from build123d import *

# Parameters (mm, degrees)
F1_DEPTH = 40
F2_W     = 40
F2_H     = 20
F3_DEPTH = 40.001
F4_R     = 5


with BuildPart() as f1:
    # F0 (on Right) → F1 (new body)
    with BuildSketch(Plane.YZ):
        Polygon((-151.999998, 380), (-184, 0), (-143.858423, 0), (-137.725254, 72.831372), (148.000002, 72.831372), (148.000002, 0), (188.000002, 0), (188.000002, 680), (163.722336, 680), (148.000002, 380), align=None)
        Polygon((148.000002, 112.831372), (-134.356833, 112.831372), (-115.226841, 340), (148.000002, 340), align=None, mode=Mode.SUBTRACT)
    extrude(amount=F1_DEPTH)

    # F2 (on face) → F3 (cut, through all)
    with BuildSketch(Plane.YZ.offset(40)):
        with Locations((-14.652766, 102.831372)):
            Rectangle(F2_W, F2_H)
    extrude(amount=-F3_DEPTH, mode=Mode.SUBTRACT)

    # F4
    f4_edges = [f1.edges().sort_by_distance(p)[0] for p in [
        (40, -167.999999, 190),
        (40, -1.999998, 380),
        (40, -163.929211, 0),
        (40, 155.861169, 530),
        (40, -140.791838, 36.415686),
        (40, 175.861169, 680),
        (40, 5.137374, 72.831372),
        (40, 188.000002, 340),
        (40, 148.000002, 36.415686),
        (40, 168.000002, 0),
        (40, -84.504799, 112.831372),
        (40, -34.652766, 102.831372),
        (40, -14.652766, 92.831372),
        (40, 5.347234, 102.831372),
        (40, 76.673618, 112.831372),
        (40, 148.000002, 226.415686),
        (40, 16.38658, 340),
        (40, -124.791837, 226.415686),
        (0, -167.999999, 190),
        (0, -1.999998, 380),
        (0, -163.929211, 0),
        (0, 155.861169, 530),
        (0, -140.791838, 36.415686),
        (0, 175.861169, 680),
        (0, 5.137374, 72.831372),
        (0, 188.000002, 340),
        (0, 148.000002, 36.415686),
        (0, 168.000002, 0),
        (0, -84.504799, 112.831372),
        (0, -34.652766, 102.831372),
        (0, -14.652766, 92.831372),
        (0, 5.347234, 102.831372),
        (0, 76.673618, 112.831372),
        (0, 148.000002, 226.415686),
        (0, 16.38658, 340),
        (0, -124.791837, 226.415686),
    ]]
    fillet(f4_edges, radius=F4_R)


solid = f1.part
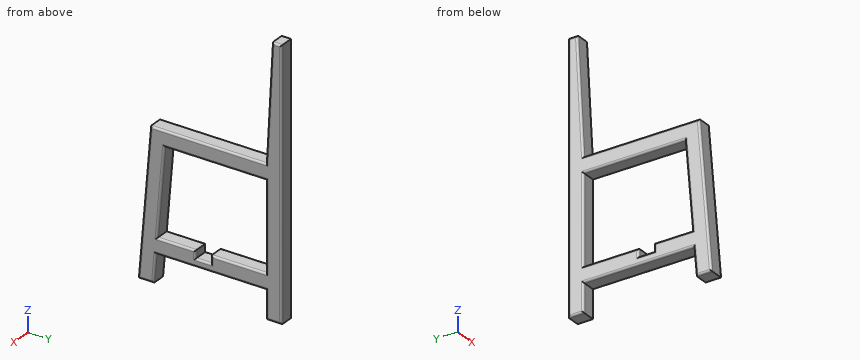
Check sheet for the modelled part. Datum: model origin and axes. Units: mm. Coordinates: 2 decimals unless noted, no trailing zeros. Write each loop counter-clockwise with the first axis right and the second up, starting at its lowest first coordinate (ties: lowest second). Pieces come first, ordered by that corner, then holes.
Item 1: Cross-section at A-A on y = 69. Record the boundary of the cut face in (x, z), then the cut area to 3 significant figures.
Numbers:
outline: (0, 77.83) arc R5 ccw to (5, 72.83) - (35, 72.83) arc R5 ccw to (40, 77.83) - (40, 107.83) arc R5 ccw to (35, 112.83) - (5, 112.83) arc R5 ccw to (0, 107.83) - close; (0, 345) arc R5 ccw to (5, 340) - (35, 340) arc R5 ccw to (40, 345) - (40, 375) arc R5 ccw to (35, 380) - (5, 380) arc R5 ccw to (0, 375) - close
area: 3,160 mm2
Item 2: Depth check by flat-ended pin: pin 1 Ø10 at (x, y) = (16, 84) entering from +Z; pin 2 Ø24 at (x, z) = (15, 49) entering from -Y; pin 3 Ø24 at (x, z) = (14.5, 258) entering from -Y. Enter the tip coordinate at first touch or a pass-through.
Numbers:
pin 1: stops at z = 380
pin 2: stops at y = -180.88
pin 3: stops at y = -163.28
Item 3: Scan lines: probe 1 along Z at (x, y) = (35, -28); probe 2 along Z at (x, y) = (9, -88.5); probe 3 along Y at (x, z) = (20, 379). Record each from-to range of solid material in increasing order.
Numbers:
probe 1: z = 72.83 to 92.83, 340 to 380
probe 2: z = 72.83 to 112.83, 340 to 380
probe 3: y = -152.08 to 188
Item 4: Cross-section at B-B on x = 22.5. Record the boundary of the cut face in (y, z).
Numbers:
outline: (-184, 0) - (-143.86, 0) - (-137.73, 72.83) - (148, 72.83) - (148, 0) - (188, 0) - (188, 680) - (163.72, 680) - (148, 380) - (-152, 380) - close; hole (-134.36, 112.83) - (-34.65, 112.83) - (-34.65, 92.83) - (5.35, 92.83) - (5.35, 112.83) - (148, 112.83) - (148, 340) - (-115.23, 340) - close
